The listing builds one solid part. Answer for the finished solid, in the listing's coordinates (mm). Face numbers are marked on the shaded views. A direction names the side the tool comes from. Coordinates: 2 decimals unless noted, no trailing zeros. Write each loop counter-clockwise with the first axis right and the second up, starting at its lowest first coordinate (ties: lowest second). Pieces come first, ordered by that corner, then holes.
from build123d import *

# Parameters (mm, degrees)
SKETCH1_W           = 118
SKETCH1_H           = 52
BOSS_EXTRUDE1_DEPTH = 2.5
SKETCH2_W           = 118
SKETCH2_H           = 52
SKETCH2_W_2         = 113
SKETCH2_H_2         = 47
EXTRUDE_THIN1_DEPTH = 47
FILLET1_R           = 10
CUT_EXTRUDE1_DEPTH  = 42.5
SKETCH5_R           = 1.7
CUT_EXTRUDE2_DEPTH  = 6


with BuildPart() as part:
    # Sketch1 → Boss-Extrude1 (new body)
    with BuildSketch(Plane(origin=(0, 0, 0), x_dir=(1, 0, 0), z_dir=(0, 1, 0))):
        with Locations((6.893384754, 6.527166983)):
            Rectangle(SKETCH1_W, SKETCH1_H)
    extrude(amount=BOSS_EXTRUDE1_DEPTH)

    # Sketch2 → Extrude-Thin1 (add)
    with BuildSketch(Plane(origin=(0, 2.5, 0), x_dir=(1, 0, 0), z_dir=(0, 1, 0))):
        with Locations((6.893384754, 6.527166983)):
            Rectangle(SKETCH2_W, SKETCH2_H)
        with Locations((6.893384754, 6.527166983)):
            Rectangle(SKETCH2_W_2, SKETCH2_H_2, mode=Mode.SUBTRACT)
    extrude(amount=EXTRUDE_THIN1_DEPTH)

    # Fillet1
    fillet1_edges = [part.edges().sort_by_distance(p)[0] for p in [
        (-49.606615246, 26, 16.972833017),
        (63.393384754, 26, 16.972833017),
        (63.393384754, 26, -30.027166983),
        (-49.606615246, 26, -30.027166983),
    ]]
    fillet(fillet1_edges, radius=FILLET1_R)

    # Sketch3 → Cut-Extrude1 (cut)
    with BuildSketch(Plane(origin=(65.893384754, 0, 0), x_dir=(0, 0, -1), z_dir=(1, 0, 0))):
        with BuildLine():
            Line((-4.831942317, 49.5), (17.886276283, 49.5))
            ThreePointArc((17.886276283, 49.5), (6.527166983, 38.1408907), (-4.831942317, 49.5))
        make_face()
    extrude(amount=-CUT_EXTRUDE1_DEPTH, mode=Mode.SUBTRACT)

    # Sketch5 → Cut-Extrude2 (cut)
    with BuildSketch(Plane(origin=(0, 49.5, 0), x_dir=(1, 0, 0), z_dir=(0, 1, 0))):
        with Locations(Location((-48.924634731, -16.290852502, 0), (0, 0, 270))):
            Circle(SKETCH5_R)
        with Locations(Location((-48.924634731, 29.345186468, 0), (0, 0, 90))):
            Circle(SKETCH5_R)
        with Locations(Location((62.711404239, -16.290852502, 0), (0, 0, 90))):
            Circle(SKETCH5_R)
        with Locations(Location((62.711404239, 29.345186468, 0), (0, 0, 270))):
            Circle(SKETCH5_R)
    extrude(amount=-CUT_EXTRUDE2_DEPTH, mode=Mode.SUBTRACT)


solid = part.part
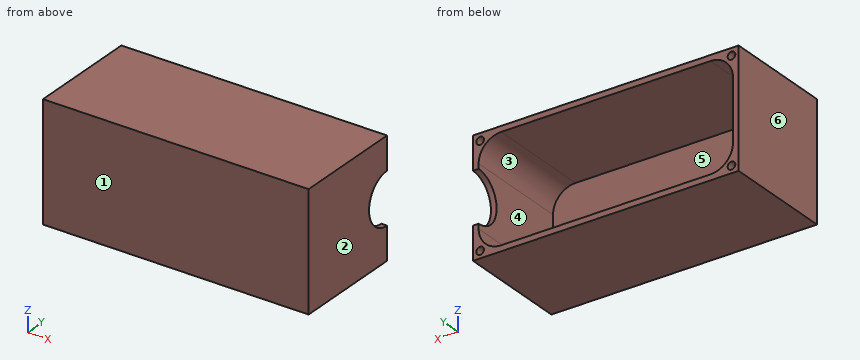
1. Section D-D on y = 40.5 is taken. Give the vertices of the cut face in (x, z), then the cut area to 3 significant figures.
Results found:
outline: (-52.11, -32.53) - (65.89, -32.53) - (65.89, -13.46) - (63.39, -13.46) - (63.39, -20.03) arc R10 cw to (53.39, -30.03) - (-39.61, -30.03) arc R10 cw to (-49.61, -20.03) - (-49.61, 6.97) arc R10 cw to (-39.61, 16.97) - (53.39, 16.97) arc R10 cw to (63.39, 6.97) - (63.39, 0.4) - (65.89, 0.4) - (65.89, 19.47) - (-52.11, 19.47) - close
area: 876 mm2
2. Section A-A on y = 17 is taken. Give the vertices of the cut face in (x, z), then the cut area to 3 significant figures.
Results found:
outline: (-52.11, -32.53) - (65.89, -32.53) - (65.89, 19.47) - (-52.11, 19.47) - close; hole (-49.61, -20.03) arc R10 ccw to (-39.61, -30.03) - (53.39, -30.03) arc R10 ccw to (63.39, -20.03) - (63.39, 6.97) arc R10 ccw to (53.39, 16.97) - (-39.61, 16.97) arc R10 ccw to (-49.61, 6.97) - close
area: 911 mm2
3. Flat-ended cylindrical pins translate along their axes: P1, Ø3, axis at x = 62.71, z = 16.29, coming from the -Y side; P2, Ø14, axis at x = -5.5, z = -12, coming from the +Y side; P3, Ø2, axis at x = 62.71, z = -29.35, coming from the +Y side. Find the tip coordinate at first contact, or state that the pin passes through.
Results found:
P1: stops at y = 0
P2: stops at y = 2.5
P3: stops at y = 43.5
4. Find the intervals of material crossed by L1, parallel to X at y = 36, z = -7.5; L2, parallel to Z at x = -17.5, y = 23; L3, parallel to Y at x = 5, z = 3, in increasing order.
Results found:
L1: x = -52.11 to -49.61, 63.39 to 65.89
L2: z = -32.53 to -30.03, 16.97 to 19.47
L3: y = 0 to 2.5
5. A tool of negligible diameter and unlimited length cuts with its end or side. For the marked faces 5 and 6, from which of +Z, -Z, +X, -X, +Y, -Y can it reach the whole face along a straight path? Write none if from no direction.
Results found:
face 5: +Y
face 6: +Z, -Z, -X, +Y, -Y
6. Section C-C on z = 3.5 is taken. Give the vertices of the cut face in (x, y).
Results found:
outline: (-52.11, 0) - (65.89, 0) - (65.89, 44.16) - (63.39, 44.16) - (63.39, 2.5) - (-49.61, 2.5) - (-49.61, 49.5) - (-52.11, 49.5) - close
7. Section B-B on x = 37.5 is taken. Give the vertices of the cut face in (y, z), then the cut area to 3 significant figures.
Results found:
outline: (0, -32.53) - (49.5, -32.53) - (49.5, -30.03) - (2.5, -30.03) - (2.5, 16.97) - (49.5, 16.97) - (49.5, 19.47) - (0, 19.47) - close
area: 365 mm2
8. For a pull along X with two mould halves and no side action, classify the marked faces 1, 2, 3 and 4 as pulls with the +X half, pulls with the -X half, needs draft (parallel to the pull), parting line crosses it, or undercut.
Results found:
face 1: needs draft
face 2: pulls with the +X half
face 3: undercut
face 4: undercut
